from build123d import *

# Parameters (mm, degrees)
SKETCH_1_W      = 64.7
SKETCH_1_H      = 33.2
EXTRUDE_1_DEPTH = 1.6
SKETCH_2_W      = 64.7
SKETCH_2_H      = 33.2
SKETCH_2_W_2    = 61.5
SKETCH_2_H_2    = 30
EXTRUDE_2_DEPTH = 95
SKETCH_4_W      = 1.6
SKETCH_4_H      = 1.6
EXTRUDE_3_DEPTH = 60


with BuildPart() as part:
    # Эскиз1 → Бобышка-Вытянуть1 (new body)
    with BuildSketch(Plane(origin=(0, 0, 0), x_dir=(1, 0, 0), z_dir=(0, 1, 0))):
        Rectangle(SKETCH_1_W, SKETCH_1_H)
    extrude(amount=EXTRUDE_1_DEPTH)

    # Эскиз2 → Бобышка-Вытянуть2 (add)
    with BuildSketch(Plane(origin=(0, 1.6, 0), x_dir=(1, 0, 0), z_dir=(0, 1, 0))):
        Rectangle(SKETCH_2_W, SKETCH_2_H)
        Rectangle(SKETCH_2_W_2, SKETCH_2_H_2, mode=Mode.SUBTRACT)
    extrude(amount=EXTRUDE_2_DEPTH)

    # Эскиз4 → Бобышка-Вытянуть3 (add)
    with BuildSketch(Plane(origin=(0, 1.6, 0), x_dir=(1, 0, 0), z_dir=(0, 1, 0))):
        with Locations((-29.95, 2.2)):
            Rectangle(SKETCH_4_W, SKETCH_4_H)
        with Locations((29.95, -1.4)):
            Rectangle(SKETCH_4_W, SKETCH_4_H)
        with Locations((-29.95, -1.4)):
            Rectangle(SKETCH_4_W, SKETCH_4_H)
        with Locations((29.95, 2.2)):
            Rectangle(SKETCH_4_W, SKETCH_4_H)
    extrude(amount=EXTRUDE_3_DEPTH)


solid = part.part
Source: CAD feature listing. Evaluate the final solid. Frame: model axes, mm. A direction names the side the tool comes from. Give positions to 0.01 mm unless a question says otherwise; leave off trailing zeros. Write each loop counter-clockwise with the first axis right and the second up, starting at its lowest first coordinate (ties: lowest second). Pieces come first, ordered by that corner, then holes. Notation, with made-up numbers: (-38, -29.75) -> (-11, -29.75) arc R37 cw to (-11, 7.25) -> close; hole circle Ø8 at (-13, 32). An arc over 180 degrees is marked (long way). Write item = value, one per line.
Q1. Mould query, pull axis Z, two halves, no side actions, for faces 1 (the face through (-32.35, 48, 0)), 2 (the face through (0, 48, 16.6)), 3 (the face through (0, 48, -16.6)), 4 (the face through (0, 48, 15)). Classes: +Z half, -Z half, draft (parallel to the pull), parting line (faces both ways), or undercut.
Here are the results:
face_1 = draft
face_2 = +Z half
face_3 = -Z half
face_4 = undercut
Q2. First-contact query: pin 1 (1.5 mm diameter, centred on x = -9.5, z = -9, fed in from +Y); pin 2 (1.3 mm diameter, centred on x = -30, z = -2.5, fed in from +Y). Flat tips, straight axial feed; report the tip coordinate or a pass-through.
Here are the results:
pin_1 = 1.6
pin_2 = 61.6
Q3. Cut plane C-C on x = 5. Return loops of the section in (y, z).
Here are the results:
outline = (0, -16.6) -> (96.6, -16.6) -> (96.6, -15) -> (1.6, -15) -> (1.6, 15) -> (96.6, 15) -> (96.6, 16.6) -> (0, 16.6) -> close
Q4. Cut plane A-A on y = 10.5. Return loops of the section in (x, z), then the cut area to 3 significant figures.
Here are the results:
outline = (-32.35, -16.6) -> (32.35, -16.6) -> (32.35, 16.6) -> (-32.35, 16.6) -> close; hole (-30.75, -15) -> (30.75, -15) -> (30.75, -3) -> (29.15, -3) -> (29.15, -1.4) -> (30.75, -1.4) -> (30.75, 0.6) -> (29.15, 0.6) -> (29.15, 2.2) -> (30.75, 2.2) -> (30.75, 15) -> (-30.75, 15) -> (-30.75, 2.2) -> (-29.15, 2.2) -> (-29.15, 0.6) -> (-30.75, 0.6) -> (-30.75, -1.4) -> (-29.15, -1.4) -> (-29.15, -3) -> (-30.75, -3) -> close
area = 313 mm²
Q5. Cut plane B-B on z = 11. Return loops of the section in (x, y), then the cut area to 3 significant figures.
Here are the results:
outline = (-32.35, 0) -> (32.35, 0) -> (32.35, 96.6) -> (30.75, 96.6) -> (30.75, 1.6) -> (-30.75, 1.6) -> (-30.75, 96.6) -> (-32.35, 96.6) -> close
area = 408 mm²
Q6. Line query: line 1 (Z direction, x = -0.5, y = 4.5); line 2 (X direction, y = 27, z = 2); line 3 (Z direction, x = 30.5, y = 8). Output: solid intervals per line, ascending. Write a range as from..to.
Here are the results:
line_1 = -16.6..-15, 15..16.6
line_2 = -32.35..-29.15, 29.15..32.35
line_3 = -16.6..-15, -3..-1.4, 0.6..2.2, 15..16.6
Q7. Reachability of faces 5 (the face through (0, 48, -15)), 6 (the face through (0, 0, 0)) from +Z, -Z, +X, -X, +Y, -Y: full face, straight path, thin tool, end or side. Return the list, or none.
Here are the results:
face_5 = +Y
face_6 = +Z, -Z, +X, -X, -Y
